Source: CAD feature listing. Evaluate the final solid. Frame: model axes, mm. Face numbers are marked on the shaded views. A direction names the side the tool comes from. Give positions to 0.01 mm unless a question says otherwise; leave off trailing zeros. Order: outer loops, then holes, each group sorted by start corner. A loop starts at its lowest first (then second) coordinate and runs counter-clockwise, first axis right, second up.
1) Section B-B, the plane z = 64.5. Return loops of the section in (x, y).
2) First-contact query: P1, Ø4, axis at x = -33, y = -8.5, coming from the +Z side; P2, Ø2, axis at y = -17.5, z = -58.5, coming from the +X side; P3, Ø3, axis at x = 18.5, z = 0.5, coming from the -Y side. Flat tips, straight axial feed; report the tip coordinate or a pass-through.
3) Section C-C, the plane z = 0. Give the number of separate pieces and of enclosed holes in the cut face, plus the area to 3 significant figures.
4) Draft query along Z for the marked faces 1, 2 and 3. Return one class per face: released by +Z, released by -Z, zero draft, split by the parting line, or undercut.
5) Material intervals for line 1 (Z direction, x = 0, y = -29.4) (3 decimals); line 2 (X direction, y = -29, z = -44); line 3 (Z direction, x = 0, y = -31) (3 decimals), sorted ascending.
6) Section A-A, the plane x = -66. Return loops of the section in (y, z), plus the area to 3 significant figures.
7) Section D-D, the plane x = 67.31. Return loops of the section in (y, z).
8) Access query for the marked faces 4 and 5. Directions: +Z, -Z, +X, -X, +Y, -Y. A direction counts if a zero-diameter tool reaches every point of the face in a straight line with its end or side. Return the directions, or none.
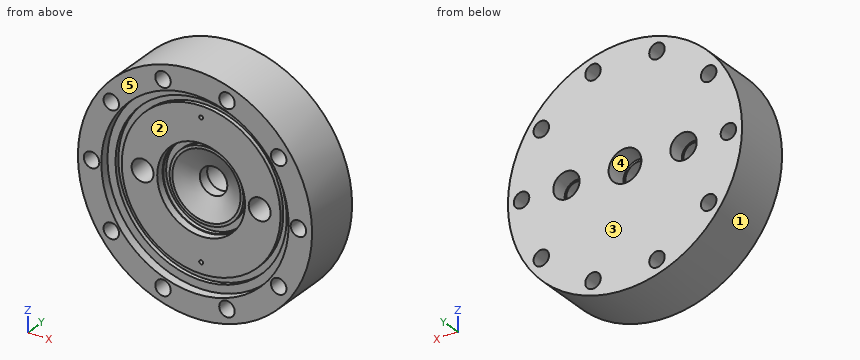
```python
from build123d import *

# Parameters (mm, degrees)
F_3_8_NPT_TAPPED_HOLE1_AT_2_COUNT = 2
F_3_8_NPT_TAPPED_HOLE1_AT_2_PITCH = 76.2
F_3_8_CLEARANCE_HOLE2_D           = 10.0838
CIRPATTERN1_COUNT                 = 10
SKETCH18_R                        = 1.27
CUT_EXTRUDE2_DEPTH                = 3.302


with BuildPart() as part:
    # Sketch1 → Revolve1 (revolve)
    with BuildSketch(Plane.XY):
        Polygon((0, 0), (-76.2, 0), (-76.2, -38.1), (-60.96, -38.1), (-60.96, -32.258), (-55.7149, -32.258), (-55.7149, -29.5656), (-51.6509, -29.5656), (-51.6509, -32.258), (-28.575, -32.258), (-28.575, -27.178), (-28.0924, -27.178), (-28.0924, -24.4856), (-24.0284, -24.4856), (-24.0284, -27.178), (-22.225, -27.178), (0, -15.85722), align=None)
    revolve(axis=Axis((0, 0, 0), (0, -1, 0)))

    # Sketch3 → 1/2 NPT Tapped Hole1 (revolve, cut)
    with BuildSketch(Plane(origin=(0, 0, 0), x_dir=(0, 0, 1), z_dir=(1, 0, 0))):
        Polygon((0, 0), (0, 38.1), (8.9281, 38.1), (8.9281, 13.462), (10.261665792, 13.462), (10.6647361, 0), align=None)
    revolve(axis=Axis((0, 6.35, 0), (0, -1, 0)), mode=Mode.SUBTRACT)

    # Sketch5 → 3/8 NPT Tapped Hole1 (revolve, cut)
    with BuildSketch(Plane(origin=(-38.1, 0, 0), x_dir=(0, 0, 1), z_dir=(1, 0, 0))):
        Polygon((0, 0), (0, 38.1), (7.1374, 38.1), (7.1374, 10.414), (8.263205494, 10.414), (8.5750146, 0), align=None)
    f_3_8_npt_tapped_hole1 = revolve(axis=Axis((-38.1, 6.35, 0), (0, -1, 0)), mode=Mode.SUBTRACT)

    # 3/8 NPT Tapped Hole1 at 2: 3/8 NPT Tapped Hole1 ×2
    with Locations(*[(i * F_3_8_NPT_TAPPED_HOLE1_AT_2_PITCH, 0, 0) for i in range(1, F_3_8_NPT_TAPPED_HOLE1_AT_2_COUNT)]):
        add(f_3_8_npt_tapped_hole1, mode=Mode.SUBTRACT)

    # 3/8 Clearance Hole2 (through all)
    with Locations(Plane(origin=(67.31, 0, 0), x_dir=(1, 0, 0), z_dir=(0, 1, 0))):
        with Locations((0, 0)):
            f_3_8_clearance_hole2 = Hole(F_3_8_CLEARANCE_HOLE2_D / 2)

    # CirPattern1: 3/8 Clearance Hole2 ×10 about axis
    cirpattern1_axis = Axis((0, 0, 0), (0, 1, 0))
    for i in range(1, CIRPATTERN1_COUNT):
        add(f_3_8_clearance_hole2.rotate(cirpattern1_axis, i * 360 / CIRPATTERN1_COUNT), mode=Mode.SUBTRACT)

    # Sketch18 → Cut-Extrude2 (cut)
    with BuildSketch(Plane.XZ.offset(32.258)):
        with Locations((0, 44.45)):
            Circle(SKETCH18_R)
        with Locations((0, -44.45)):
            Circle(SKETCH18_R)
    extrude(amount=-CUT_EXTRUDE2_DEPTH, mode=Mode.SUBTRACT)


solid = part.part
```
From the geometry:
1. outline: (-40.57, -38.1) - (-25.82, -38.1) - (-25.82, 0) - (-40.57, 0) - close; (-15.78, -38.1) - (15.78, -38.1) - (15.78, 0) - (-15.78, 0) - close; (25.82, -38.1) - (40.57, -38.1) - (40.57, 0) - (25.82, 0) - close
2. P1: stops at z = 69.61
2. P2: stops at x = 50
2. P3: stops at y = -26.05
3. separate pieces: 6
3. enclosed holes: 0
3. area: 2,400 mm2
4. face 1: split by the parting line
4. face 2: undercut
4. face 3: zero draft
5. line 1: z = -76.2 to -45.72, -43.18 to -28.575, 28.575 to 43.18, 45.72 to 76.2
5. line 2: x = -62.21 to -56.85, -52.06 to -1.19, 1.19 to 52.06, 56.85 to 62.21
5. line 3: z = -76.2 to -55.715, -51.651 to -45.72, -43.18 to -28.575, 28.575 to 43.18, 45.72 to 51.651, 55.715 to 76.2
6. outline: (-38.1, -38.08) - (0, -38.08) - (0, -4.87) - (-38.1, -4.87) - close; (-38.1, 4.87) - (0, 4.87) - (0, 38.08) - (-38.1, 38.08) - close
6. area: 2,530 mm2
7. outline: (-38.1, -35.72) - (0, -35.72) - (0, -5.04) - (-38.1, -5.04) - close; (-38.1, 5.04) - (0, 5.04) - (0, 35.72) - (-38.1, 35.72) - close
8. face 4: +Y
8. face 5: +Z, -Z, +X, -X, -Y
